Geometry: final body of the model. Coordinates: model frame, mm. A direction names the side the tool comes from. Coordinates: 2 decimals unless noted, no trailing zeros. Order: outer loops, then holes, each group sorted by start corner. A loop starts at its lowest first (then second) coordinate and runs counter-clockwise, first axis right, second up. Notation, with made-up numbers: (71, -19.5) - (93, -19.5) arc R9 cw to (93, -8.5) - close; hole circle Ø5 at (18, -40). An arc over 180 degrees is marked (long way). Use one line per item in the form item = value. Start each with the question number.
```python
from build123d import *

# Parameters (mm, degrees)
F0_W     = 42.3
F0_H     = 42.3
F1_DEPTH = 46.3
F2_SIZE  = 5
F3_R     = 11
F4_DEPTH = 2
F5_R     = 2.5
F6_DEPTH = 24
F8_D     = 3.3


with BuildPart() as f1:
    # F0 (on Front) → F1 (new body)
    with BuildSketch(Plane.XZ):
        Rectangle(F0_W, F0_H)
    extrude(amount=-F1_DEPTH)

    # F2
    f2_edges = [f1.edges().sort_by_distance(p)[0] for p in [
        (-21.15, 23.15, 21.15),
        (21.15, 23.15, 21.15),
        (-21.15, 23.15, -21.15),
        (21.15, 23.15, -21.15),
    ]]
    chamfer(f2_edges, length=F2_SIZE)

    # F3 (on face) → F4 (join)
    with BuildSketch(Plane.XZ):
        Circle(F3_R)
    extrude(amount=F4_DEPTH)

    # F5 (on face) → F6 (join)
    with BuildSketch(Plane.XZ.offset(2)):
        Circle(F5_R)
    extrude(amount=F6_DEPTH)

    # F8 (through all)
    with Locations(Plane.XZ):
        with Locations((15.5, 15.5), (-15.5, 15.5), (-15.5, -15.5), (15.5, -15.5)):
            Hole(F8_D / 2)


solid = f1.part
```
(1) Cut plane C-C on y = -10. Return the cut outline in (x, z), plus the area to 3 significant figures.
(2) Draft query along Z for faces 1 (the flat face through (-21.15, 23, 0)), 2 (the cylindrical face through (13.926, 23.474, -15.004)), 3 (the cylindrical face through (-17.024, 23.474, 14.868)), 4 (the flat face through (-18.6, 22.8, 18.7)). Return one class per face: released by +Z, released by -Z, zero draft, split by the parting line, or undercut.
(3) Cut plane A-A on z = 5.5. Return the cut outline in (x, y).
(4) Contact query for flat-ended pins moving along their axis: pin 1 Ø5.5 at (x, z) = (-15.5, 15.5) entering from -Y; pin 2 Ø2 at (x, z) = (-4, 9) entering from -Y; pin 3 Ø12 at (x, y) = (7.5, -11.5) entering from +Z. Output: stop coordinate, or through.
(5) Cut plane B-B on x = 0. Return the cut outline in (y, z).
(6) Cut plane D-D on x = 8. Return the cut outline in (y, z), plus the area to 3 significant figures.
(7) Set-up query: faces 5 (the cylindrical face through (-2.38, -0.99, -10.74)), 6 (the flat face through (0, 23, 21.15)). Return all of +Z, -Z, +X, -X, +Y, -Y with unobstructed straight access to the full face (end or side cutting, diameter ignored); none if empty.
(8) Material intervals for L1, parallel to Z at x = -15.5, y = 18.5; L2, parallel to X at y = 13, z = -15; L3, parallel to Y at x = 13, z = -7.5, sorted ascending. Write a range as from..to.
Check sheet entries:
q1.outline = circle Ø5 at (0, 0)
q1.area = 19.6 mm^2
q2.face_1 = zero draft
q2.face_2 = undercut
q2.face_3 = undercut
q2.face_4 = released by +Z
q3.outline = (-21.15, 0) - (-9.53, 0) - (-9.53, -2) - (9.53, -2) - (9.53, 0) - (21.15, 0) - (21.15, 46.3) - (-21.15, 46.3) - close
q4.pin_1 = 0
q4.pin_2 = -2
q4.pin_3 = 2
q5.outline = (-26, -2.5) - (-2, -2.5) - (-2, -11) - (0, -11) - (0, -21.15) - (46.3, -21.15) - (46.3, 21.15) - (0, 21.15) - (0, 11) - (-2, 11) - (-2, 2.5) - (-26, 2.5) - close
q6.outline = (-2, -7.55) - (0, -7.55) - (0, -21.15) - (46.3, -21.15) - (46.3, 21.15) - (0, 21.15) - (0, 7.55) - (-2, 7.55) - close
q6.area = 1,990 mm^2
q7.face_5 = -Y
q7.face_6 = +Z, +X, -X, +Y, -Y
q8.L1 = -21.15..-17.15, -13.85..13.85, 17.15..21.15
q8.L2 = -21.15..-17.07, -13.93..13.93, 17.07..21.15
q8.L3 = 0..46.3
